Source: three-view drawing plus pictorial views. Frame: mm from the lowest corner of the part. A direction names the side the tool comes from. Round coordinates to 2 decimals unless told otherwise and drop trailing zeros. Order: outer loops, then holes, each group sorted by start corner. A loop starts at its lowest first (then second) coordinate and runs counter-clockwise, first axis right, second up. Notation, with made-up numbers: M 70,72 L 80,72 A35 cw 80,105 Z; hole C 25.5,-13 d10. An arc over 180 degrees is marked long. Return JSON: item names as keys, results as strings. Group by question number.
Q1. Cut plane D-D on y = 1.25. Output: boundary loops of the cut face in (x, z), and give its area (3 significant figures).
Q2. Access query for the marked faces 1 and 2. Directions: +Z, -Z, +X, -X, +Y, -Y. A direction counts if a zero-diameter tool reaches every point of the face in a straight line with its end or side. Return the directions, or none.
Q3. Cut plane C-C on y = 4. Output: boundary loops of the cut face in (x, z) (3 decimals).
Q4. Contact query for flat-ended pins moving along their axis: pin 1 (1 mm diameter, centred on x = 3, y = 2.5, fed in from -Z); pin 2 (1 mm diameter, centred on x = 8, y = 5, fed in from -Z); pin 3 (0.7 mm diameter, centred on x = 4.5, z = 4.5, fed in from +Y); pin 4 (3 mm diameter, centred on x = 2.5, y = 5, fed in from +Z). Output: stop coordinate, or through.
Q5. Ray query, probe 1 along X at (y, z) = (1.65, 4.5); probe 2 along Y at (x, z) = (6.9, 4.5); probe 3 along Y at (x, z) = (3.5, 8.25). Return the intervals inside material, ascending.
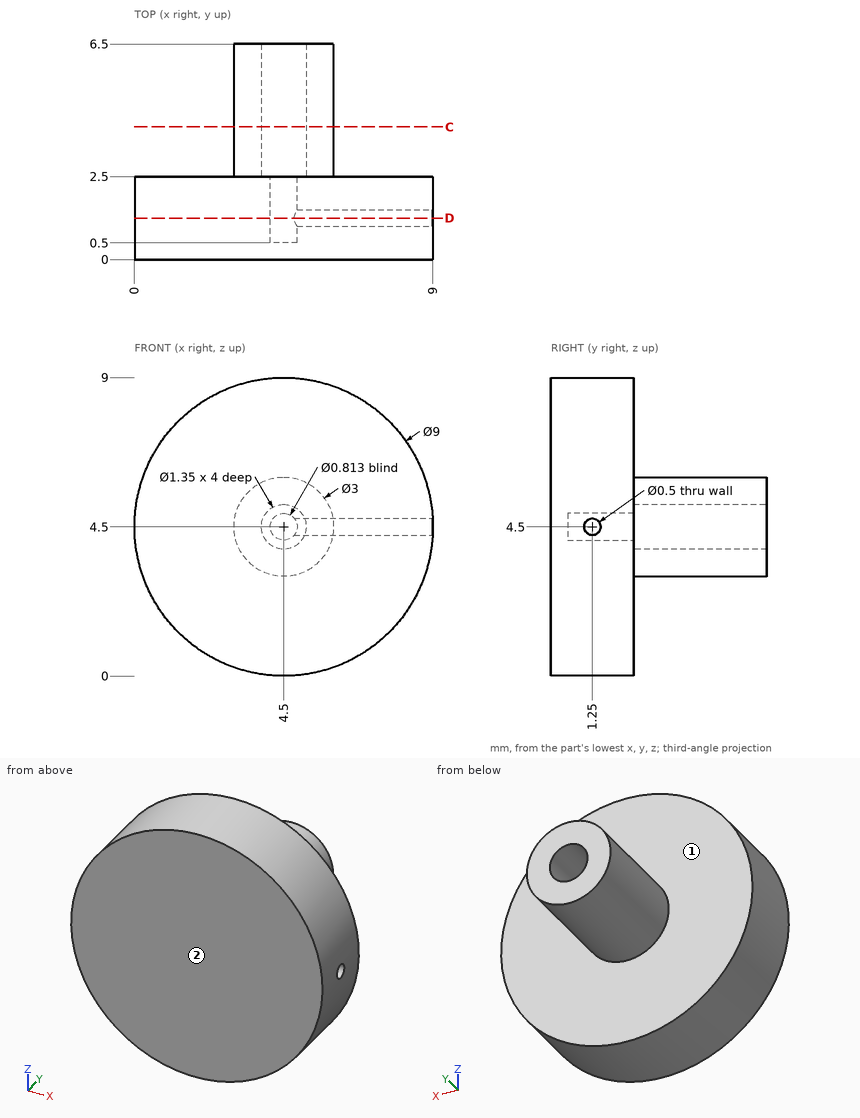
Result sheet:
{
 "1": {"outline": "M 4.82,4.25 A0.41 cw long 4.82,4.75 L 8.99,4.75 A4.5 ccw long 8.99,4.25 Z", "area": "61.0 mm²"},
 "2": {"face 1": "+Y", "face 2": "+Z, -Z, +X, -X, -Y"},
 "3": {"outline": "C 4.5,4.5 d3; hole C 4.5,4.5 d1.35"},
 "4": {"pin 1": "stops at z = 0.11", "pin 2": "passes through", "pin 3": "stops at y = 0.5", "pin 4": "stops at z = 5.91"},
 "5": {"probe 1": "x = 0 to 4.09, 4.91 to 9", "probe 2": "y = 0 to 1, 1.5 to 2.5", "probe 3": "y = 0 to 2.5"}
}
